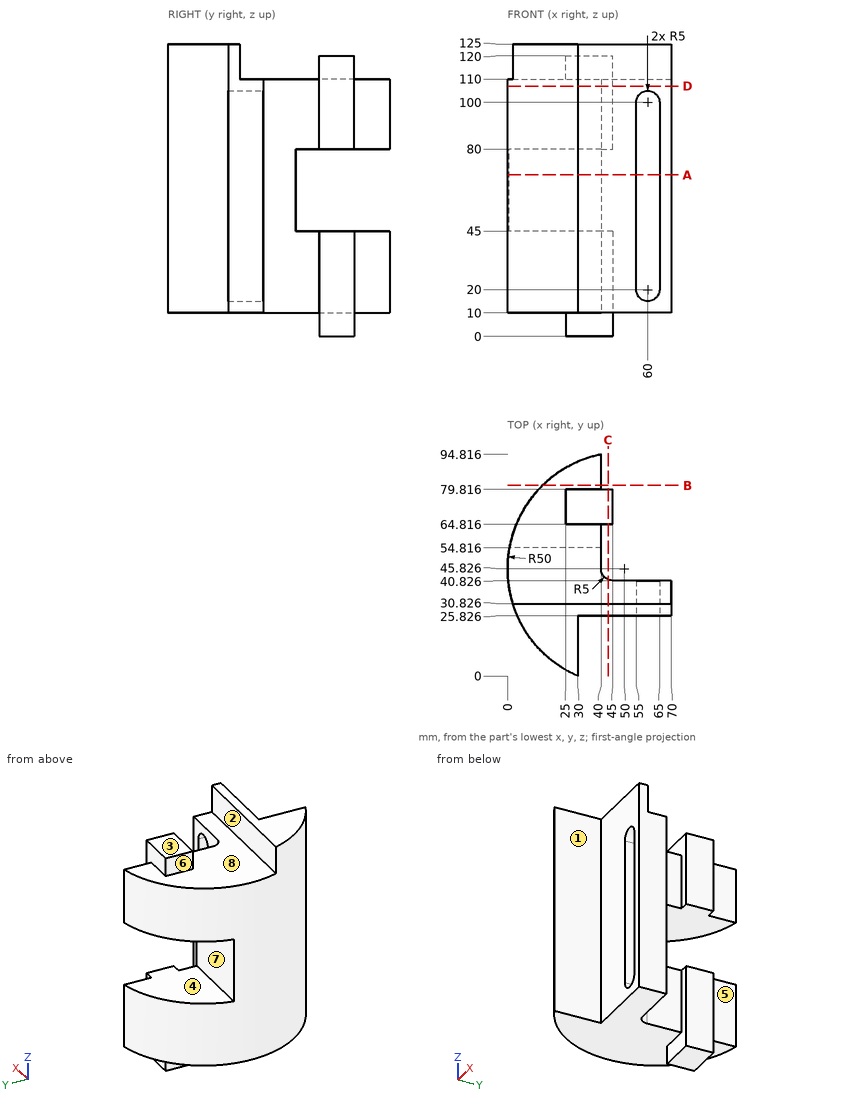
Geometry: see drawing. Coordinates: mm, zero at the bounding-box minimum. A direction names the side the tool comes from. Give positions to 0.01 mm unless a question says otherwise; leave off trailing zeros. Loops run counter-clockwise (first coordinate to the right, second up) from the corner with the lowest first, then second, coordinate; pieces in that order, holes last. Notation, with made-up numbers: (48.25, 68) - (77.25, 68) arc R24 cw to (77.25, 89) - close; hole circle Ø7 at (-1, 23). An arc over 180 degrees is marked (long way). Use CSV: the item, a comma, the result in double quotes. Start each with the question number.
Item 1: Mould query, pull axis Y, two halves, no side actions, for the marked faces 6, 7 and 8. Classes: pulls with the +Y half, pulls with the -Y half, needs draft (parallel to the pull), parting line crosses it, or undercut.
Item 2: Section D-D on z = 107. Return loops of the section in (x, y) (1 decimal), then the cut area to 3 significant figures.
Item 3: Contact query for flat-ended pins moving along their axis: P1, Ø3, axis at x = 56.5, y = 41.5, coming from the +Z side; P2, Ø16.5, axis at x = 39.5, y = 71.5, coming from the +Z side; P3, Ø6, axis at x = 37.5, z = 31, coming from the -Y side; P4, Ø8, axis at x = 52.5, y = 69.5, coming from the -Z side. Output: stop coordinate, or through.
Item 4: Section C-C on x = 43. Return loops of the section in (y, z) (1 decimal).
Item 5: Section B-B on y = 81.5. Return loops of the section in (x, z), then the cut area to 3 significant figures.
Item 6: Section A-A on z = 69. Return loops of the section in (x, y) (1 decimal).
Item 7: Line query: line 1 (Z direction, x = 16, y = 56); line 2 (Z direction, x = 24, y = 53); line 3 (X direction, y = 37, z = 58.5) (1 decimal). Output: solid intervals per line, ascending.
Item 8: Reachability of the marked faces 1, 2, 3, 4 and 5 from +Z, -Z, +X, -X, +Y, -Y: full face, straight path, thin tool, end or side. Return the list, or none.
Ans:
1,face 6,"needs draft"
1,face 7,"pulls with the +Y half"
1,face 8,"undercut"
2,outline,"(30, 0) - (30, 25.8) - (70, 25.8) - (70, 40.8) - (45, 40.8) arc R5 cw to (40, 45.8) - (40, 64.8) - (45, 64.8) - (45, 79.8) - (40, 79.8) - (40, 94.8) arc R50 ccw to start"
2,area,"3,190 mm2"
3,P1,"stops at z = 110"
3,P2,"stops at z = 120"
3,P3,"stops at y = 25.83"
3,P4,"passes through"
4,outline,"(25.8, 10) - (41.2, 10) - (41.2, 110) - (30.8, 110) - (30.8, 125) - (25.8, 125) - close; (64.8, 0) - (79.8, 0) - (79.8, 45) - (64.8, 45) - close; (64.8, 80) - (79.8, 80) - (79.8, 120) - (64.8, 120) - close"
5,outline,"(14.97, 10) - (40, 10) - (40, 45) - (14.97, 45) - close; (14.97, 80) - (40, 80) - (40, 110) - (14.97, 110) - close"
5,area,"1,630 mm2"
6,outline,"(0.8, 54.8) arc R50 ccw to (30, 0) - (30, 25.8) - (55, 25.8) - (55, 40.8) - (45, 40.8) arc R5 cw to (40, 45.8) - (40, 54.8) - close; (65, 25.8) - (70, 25.8) - (70, 40.8) - (65, 40.8) - close"
7,line 1,"z = 10 to 45, 80 to 110"
7,line 2,"z = 10 to 110"
7,line 3,"x = 0.8 to 55, 65 to 70"
8,face 1,"+Z, -Z, +X, -Y"
8,face 2,"+Z, +X, -X"
8,face 3,"+Z, +X, -X, +Y"
8,face 4,"+X, -X, +Y"
8,face 5,"+Z, -Z, +X, +Y"
